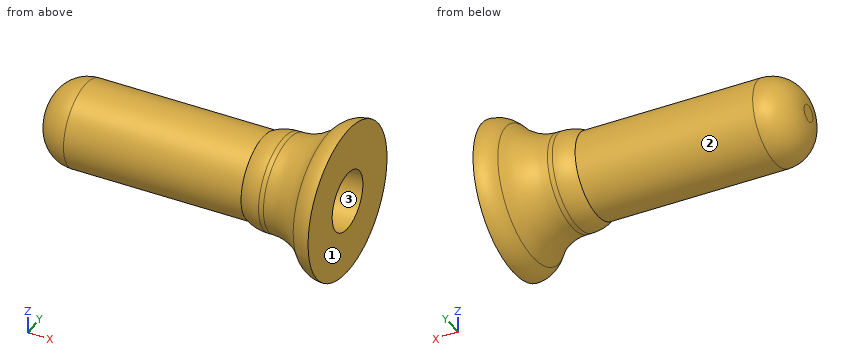
from build123d import *

# Parameters (mm, degrees)
SKETCH2_R          = 3.5
CUT_EXTRUDE1_DEPTH = 10
FILLET7_R          = 3
FILLET8_R          = 6
FILLET9_R          = 5
FILLET10_R         = 4


# Some blends are built 0.0001 mm under size
with BuildPart() as part:
    # Sketch1 → Revolve1 (revolve)
    with BuildSketch(Plane(origin=(0, 0, 0), x_dir=(1, 0, 0), z_dir=(0, 1, 0)), mode=Mode.PRIVATE) as revolve1_sk:
        Polygon((0, 0), (0, 9), (-3, 9), (-3, 5.60541789), (-10, 5.60541789), (-10, 5), (-35, 5), (-35, 0), align=None)
    revolve(revolve1_sk.sketch.rotate(Axis((-35, 0, 0), (1, 0, 0)), 180), axis=Axis((-35, 0, 0), (1, 0, 0)))

    # Sketch2 → Cut-Extrude1 (cut)
    with BuildSketch(Plane(origin=(0, 0, 0), x_dir=(0, 0, -1), z_dir=(1, 0, 0))):
        Circle(SKETCH2_R)
    extrude(amount=-CUT_EXTRUDE1_DEPTH, mode=Mode.SUBTRACT)

    # Fillet7
    fillet7_edges = [part.edges().sort_by_distance(p)[0] for p in [
        (-3, 0, -9),
    ]]
    fillet(fillet7_edges, radius=FILLET7_R - 0.0001)  # a hair under: the kernel refuses the full size

    # Fillet8
    fillet8_edges = [part.edges().sort_by_distance(p)[0] for p in [
        (-3, 0, -5.60541789),
    ]]
    fillet(fillet8_edges, radius=FILLET8_R)

    # Fillet9
    # the kernel refuses this fillet: 5 mm, written as the material it takes off along each edge
    with BuildSketch(Plane(origin=(-10, 0, 0), x_dir=(0, 0, 1), z_dir=(0, 1, 0))) as fillet9_piece_1:
        with BuildLine():
            CenterArc((0.60541789, 2.384879049), FILLET9_R, 331.51192705, 28.48807295)
            Line((5, 0), (5.60541789, 0))
            Line((5.60541789, 0), (5.60541789, 2.384879049))
        make_face()
    revolve(axis=Axis((-10, 0, 0), (1, 0, 0)), mode=Mode.SUBTRACT)

    # Fillet10
    fillet10_edges = [part.edges().sort_by_distance(p)[0] for p in [
        (-35, 0, -5),
    ]]
    fillet(fillet10_edges, radius=FILLET10_R)


solid = part.part
Here's how the part is built. I have some questions about the finished solid (model axes, mm). Face numbers are marked on the shaded views. Give positions to 0.01 mm unless a question says otherwise; leave off trailing zeros. Order: outer loops, then holes, each group sorted by start corner. A loop starts at its lowest first (then second) coordinate and runs counter-clockwise, first axis right, second up. Notation, with made-up numbers: (39, 41) -> (59, 41) arc R26 ccw to (59, 68) -> close; hole circle Ø5 at (-18.5, -5). An arc over 180 degrees is marked (long way). Use a Markdown table: item, result. Add a question column.
Item 1: If we mould it in two halves opening along Z, with no side actions, what happens to the marked faces 1, 2 and 3? For each: pulls with the +Z half, pulls with the -Z half, needs draft (parallel to the pull), parting line crosses it, or undercut.
Item 2: Imagine slicing it at A-A on x = -13. Please give me the cut outline in (y, z).
Item 3: Will these pins go through, and if not, where does the flat tip stop? pin 1 (1 mm diameter, centred on x = -17.5, y = 6, fed in from -Z); pin 2 (5 mm diameter, centred on y = -4, z = -4, fed in from -X); pin 3 (3.5 mm diameter, centred on y = 1, z = -1, fed in from +X); pin 4 (1.5 mm diameter, centred on x = -15, z = 0, fed in from +Y).
Item 4: I need wall thicknesses on line 1 (Y direction, x = -7.5, z = 0); line 2 (Y direction, x = -2.75, z = 0); line 3 (Z direction, x = -6, y = 2). Which ranges of each line are inside material? Lowest first, please.
Data:
| question | item | result |
|---|---|---|
| 1 | face 1 | needs draft |
| 1 | face 2 | parting line crosses it |
| 1 | face 3 | undercut |
| 2 | outline | circle Ø10 at (0, 0) |
| 3 | pin 1 | passes through |
| 3 | pin 2 | stops at x = -34.37 |
| 3 | pin 3 | stops at x = -10 |
| 3 | pin 4 | stops at y = 5 |
| 4 | line 1 | y = -5.61 to -3.5, 3.5 to 5.61 |
| 4 | line 2 | y = -7.41 to -3.5, 3.5 to 7.41 |
| 4 | line 3 | z = -5.33 to -2.87, 2.87 to 5.33 |
